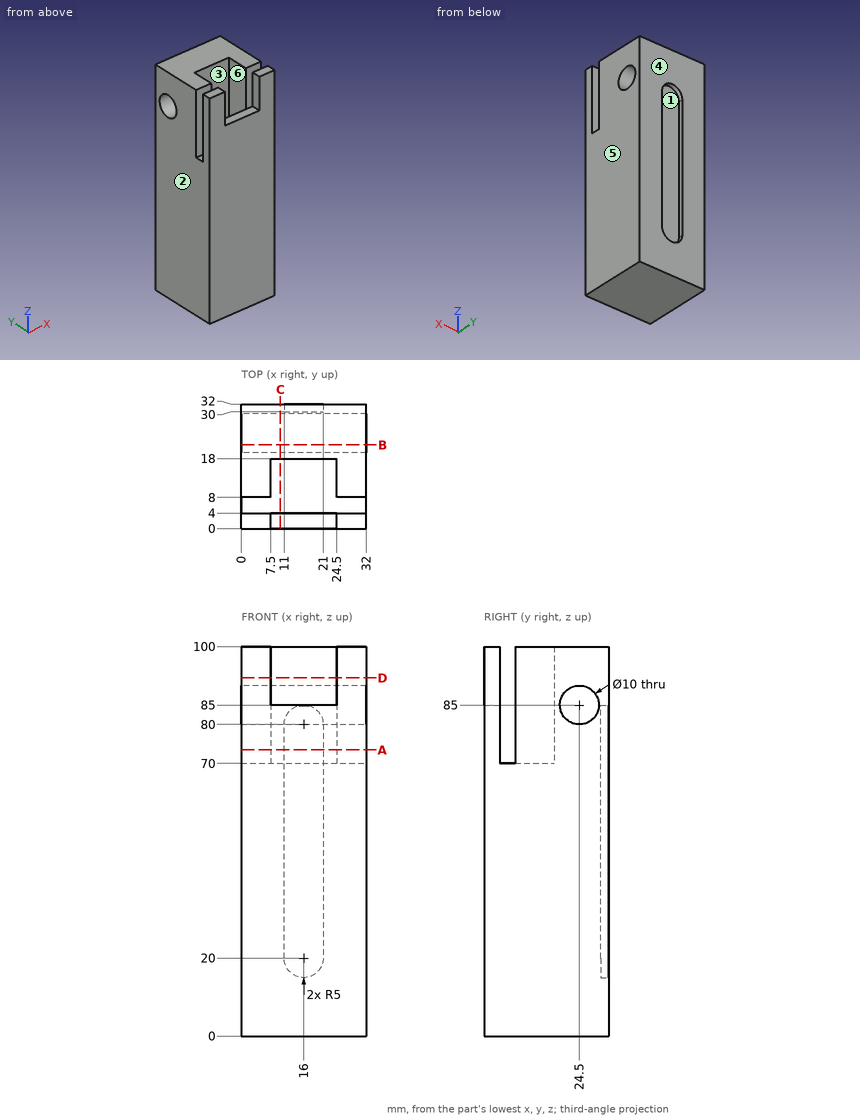
Here's the drawing with two shaded views (mm, measured from the low corner). I have some questions. A direction names the side the tool comes from. Round coordinates to 2 decimals unless told otherwise and drop trailing zeros. Loops run counter-clockwise (first coordinate to the right, second up) from the corner with the lowest first, then second, coordinate; pieces in that order, holes last. Notation, with made-up numbers: (81, -15.5) - (131, -15.5) arc R15 cw to (131, 12.5) - close; hole circle Ø10 at (79, -13). An arc over 180 degrees is marked (long way). Write item = value, one per line.
1) Imagine slicing it at C-C (x = 10). Please give me the cut outline in (y, z), and give its area (3 significant figures).
Computed:
outline = (0, 0) - (32, 0) - (32, 100) - (18, 100) - (18, 70) - (4, 70) - (4, 85) - (0, 85) - close; hole circle Ø10 at (24.5, 85)
area = 2,640 mm2
2) If we mould it in two halves opening along X, with no side actions, what happens to the marked faces 4, 5 and 6? For each: pulls with the +X half, pulls with the -X half, needs draft (parallel to the pull), parting line crosses it, or undercut.
Computed:
face_4 = needs draft
face_5 = pulls with the +X half
face_6 = undercut
3) On a 3-axis mill with a long thin cutter (end or side, diameter ignored), from which of +Z, -Z, +X, -X, +Y, -Y can I reach the whole of each face in a straight line? I mean the marked faces 1, 2 and 3. Say none if no direction works.
Computed:
face_1 = +Y
face_2 = +Z, -Z, -X, +Y, -Y
face_3 = +Z
4) Imagine slicing it at B-B (y = 21.5). Please give me the cut outline in (x, z), and give its area (3 significant figures).
Computed:
outline = (0, 0) - (32, 0) - (32, 81) - (0, 81) - close; (0, 89) - (32, 89) - (32, 100) - (0, 100) - close
area = 2,940 mm2
5) I need wall thicknesses on line 1 along Y through (x, z) = (25, 85); line 2 along Y through (x, z) = (16, 78.5); line 3 along Y through (x, z) = (25, 74.5). Which ranges of each line are inside material? Lowest first, please. Write a range as from..to.
Computed:
line_1 = 0..4, 8..19.5, 29.5..32
line_2 = 0..4, 18..30
line_3 = 0..4, 8..32
6) I'm going to push flat-ended pins straight in: P1, Ø10, axis at y = 20.5, z = 49.5, coming from the -X side; P2, Ø3, axis at x = 18, y = 2, coming from the +Z side; P3, Ø3, axis at x = 15, z = 77.5, coming from the +Y side. Where does each tip first touch, or does it pass through?
Computed:
P1 = 0
P2 = 85
P3 = 30
7) Imagine slicing it at D-D (z = 92). Please give me the cut outline in (x, y).
Computed:
outline = (0, 0) - (7.5, 0) - (7.5, 4) - (0, 4) - close; (0, 8) - (7.5, 8) - (7.5, 18) - (24.5, 18) - (24.5, 8) - (32, 8) - (32, 32) - (0, 32) - close; (24.5, 0) - (32, 0) - (32, 4) - (24.5, 4) - close
8) Imagine slicing it at A-A (z = 73.5). Please give me the cut outline in (x, y).
Computed:
outline = (0, 0) - (32, 0) - (32, 4) - (0, 4) - close; (0, 8) - (7.5, 8) - (7.5, 18) - (24.5, 18) - (24.5, 8) - (32, 8) - (32, 32) - (21, 32) - (21, 30) - (11, 30) - (11, 32) - (0, 32) - close
